Autodesk Inventor part; units mm, degrees
sketch "Esboço1" plane through (0, 0, 0) normal (0, 0, 1) x (1, 0, 0)
  line L0 (-800, -400) -> (800, -400)
  line L1 (800, -400) -> (800, 400)
  line L2 (800, 400) -> (-800, 400)
  line L3 (-800, 400) -> (-800, -400)
  line L4 (-800, -400) -> (800, 400) construction
  line L5 (800, -400) -> (-800, 400) construction
  point P0 (0, 0)
  dimension "d0" = 1600
  dimension "d1" = 800
extrude "Extrusão1" add sketch "Esboço1" along normal mid plane 30
fillet "Arredondamento1" radius 30 1 edges at (-800, 400, 0)
fillet "Arredondamento2" radius 30 1 edges at (800, 400, 0)
fillet "Arredondamento3" radius 30 1 edges at (800, -400, 0)
fillet "Arredondamento4" radius 30 1 edges at (-800, -400, 0)
sketch "Esboço3" plane through (0, 0, -15) normal (0, 0, -1) x (-1, 0, 0)
  circle A0 centre (-750, 350) radius 35.4
  circle A1 centre (-750, 350) radius 17.1
  point P0 (0, 0)
  dimension "d9" = 70.8
  dimension "d10" = 350
  dimension "d11" = 750
  dimension "d13" = 34.2
extrude "Extrusão2" cut sketch "Esboço3" against normal blind 15
mirror "Espelhar1" about plane through (0, 0, 0) normal (1, 0, 0) of "Extrusão2"
mirror "Espelhar2" about plane through (0, 0, 0) normal (0, 1, 0) of "Extrusão2", "Espelhar1"
properties part number "Sessao7_02_04_2025_999_0001" material "Madeira (Cerejeira)"
Input: part model. Units: mm. Frame: model coordinates. A direction names the side the tool comes from. Give positions to 0.01 mm unless a question says otherwise; leave off trailing zeros. Order: outer loops, then holes, each group sorted by start corner. A loop starts at its lowest first (then second) coordinate and runs counter-clockwise, first axis right, second up. Notation, with made-up numbers: M 2.5,75 L 53.5,75 A21 ccw 53.5,93 Z; hole C 69,68 d1. An arc over 180 degrees is marked long. Return JSON: item names as keys, results as strings.
1) Line query: L1, parallel to Y at x = -750, z = -8.25; L2, parallel to X at y = -350, z = -7.75; L3, parallel to X at y = 352, z = -13.25. Output: solid intervals per line, ascending. Write a range as [from, to].
Taken from the geometry:
{"L1": "y = [-400, -385.4], [-367.1, -332.9], [-314.6, 314.6], [332.9, 367.1], [385.4, 400]", "L2": "x = [-800, -785.4], [-767.1, -732.9], [-714.6, 714.6], [732.9, 767.1], [785.4, 800]", "L3": "x = [-800, -785.34], [-766.98, -733.02], [-714.66, 714.66], [733.02, 766.98], [785.34, 800]"}
2) Section query A-A on y = 350. Output: boundary loops of the cut face in (x, z).
Taken from the geometry:
{"outline": "M -800,-15 L -785.4,-15 L -785.4,0 L -767.1,0 L -767.1,-15 L -732.9,-15 L -732.9,0 L -714.6,0 L -714.6,-15 L 714.6,-15 L 714.6,0 L 732.9,0 L 732.9,-15 L 767.1,-15 L 767.1,0 L 785.4,0 L 785.4,-15 L 800,-15 L 800,15 L -800,15 Z"}
3) Mould query, pull axis Y, two halves, no side actions, for faces 3 (the face through (763.57, -360.405, -7.605)), 4 (the face through (-791.445, 390.979, -0.21)), 5 (the face through (-11, 6, -15)), 6 (the face through (-11, -400, 0)). Classes: released by +Y, released by -Y, zero draft, split by the parting line, or undercut.
Taken from the geometry:
{"face 3": "undercut", "face 4": "released by +Y", "face 5": "zero draft", "face 6": "released by -Y"}
4) Access query for faces 1 (the face through (790.979, 391.445, -0.21)), 2 (the face through (-763.57, 360.405, -7.605)). Directions: +Z, -Z, +X, -X, +Y, -Y. A direction counts if a zero-diameter tool reaches every point of the face in a straight line with its end or side. Return the directions, or none.
Taken from the geometry:
{"face 1": "+Z, -Z, +X, +Y", "face 2": "-Z"}
5) Section query B-B on x = -750. Output: boundary loops of the cut face in (y, z).
Taken from the geometry:
{"outline": "M -400,-15 L -385.4,-15 L -385.4,0 L -367.1,0 L -367.1,-15 L -332.9,-15 L -332.9,0 L -314.6,0 L -314.6,-15 L 314.6,-15 L 314.6,0 L 332.9,0 L 332.9,-15 L 367.1,-15 L 367.1,0 L 385.4,0 L 385.4,-15 L 400,-15 L 400,15 L -400,15 Z"}
